Source: three-view drawing plus pictorial views. Frame: mm from the lowest corner of the part. Coordinates: 2 decimals unless noted, no trailing zeros. Write each loop counter-clockwise with the first axis right and the second up, starting at its lowest first coordinate (ties: lowest second). Pieces come first, ordered by that corner, then holes.
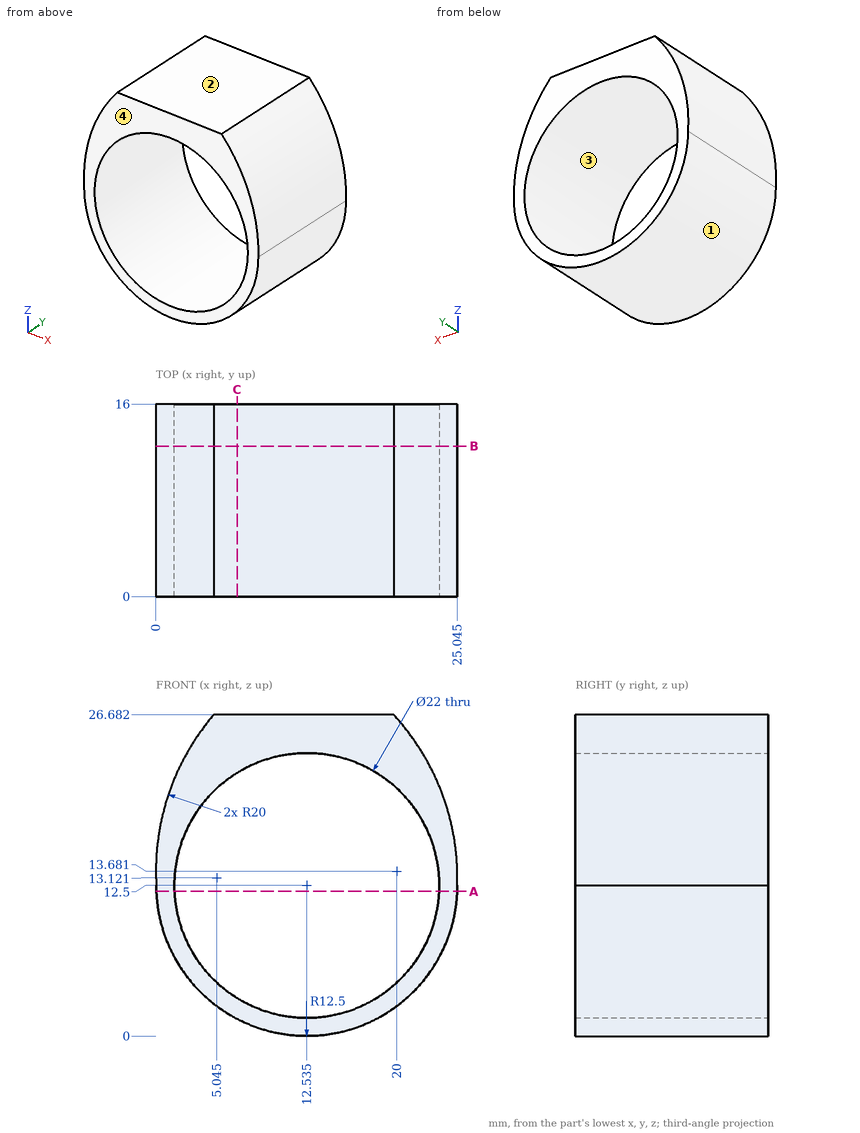
Item 1: Material intervals for line 1 (X direction, y = 12.5, z = 20.5) (1 decimal); line 2 (X direction, y = 1.25, z = 5.25); line 3 (Z direction, x = 18.75, y = 12.75) (1 decimal), sorted ascending.
Item 2: Pull-direction query (Z, two-part tool) for the marked faces 1, 2, 3 and 4; classes: released by +Z, released by -Z, zero draft, split by the parting line, or undercut.
Item 3: Section query B-B, the plane y = 12.5. Return loops of the section in (x, z) (1 decimal).
Item 4: Pin query (flat end, axial travel): pin 1 Ø5 at (y, z) = (8.5, 23) entering from -X; pin 2 Ø1.5 at (x, y) = (11, 5.5) entering from -Z (1 decimal); pin 3 Ø3 at (y, z) = (13, 18.5) entering from -X. Return the tip coordinate at first contact, or that it passes through.
Item 5: Section query A-A, the plane z = 12. Return loops of the section in (x, y) (1 decimal).
Item 6: Section query C-C, the plane x = 6.75. Return loops of the section in (y, z).
The answers:
1. line 1: x = 1.2 to 5, 20.1 to 23.6
1. line 2: x = 2.35 to 4.26, 20.81 to 22.72
1. line 3: z = 1.7 to 3.4, 21.6 to 26.7
2. face 1: released by -Z
2. face 2: released by +Z
2. face 3: undercut
2. face 4: zero draft
3. outline: (0, 12.5) arc R12.5 ccw to (25, 12.5) arc R20 ccw to (19.7, 26.7) - (4.8, 26.7) arc R20 ccw to start; hole circle Ø22 at (12.5, 12.5)
4. pin 1: stops at x = 1.2
4. pin 2: stops at z = 0
4. pin 3: stops at x = 0.28
5. outline: (0, 0) - (1.5, 0) - (1.5, 16) - (0, 16) - close; (23.5, 0) - (25, 0) - (25, 16) - (23.5, 16) - close
6. outline: (0, 1.42) - (16, 1.42) - (16, 3.14) - (0, 3.14) - close; (0, 21.86) - (16, 21.86) - (16, 26.68) - (0, 26.68) - close
